CAD build for the part. Positions are in the model's coordinates, mm. Coordinates: 2 decimals unless noted, no trailing zeros. Order: outer loops, then holes, each group sorted by start corner. A loop starts at its lowest first (then second) coordinate and runs counter-clockwise, first axis right, second up. Notation, with made-up numbers: (32.5, 22.5) - (37.5, 22.5) arc R21 ccw to (37.5, 42.5) - close; hole circle Ø1 at (-25.5, 85). An arc over 180 degrees is marked (long way). Return JSON: item names as keys, results as strings.
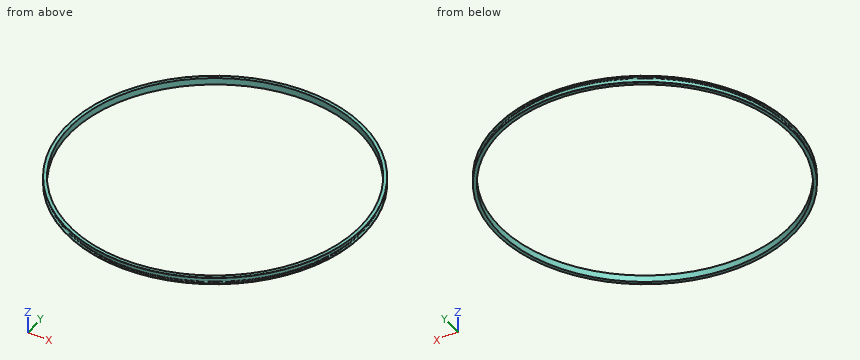
from build123d import *


with BuildPart() as part:
    # Sketch1 → Revolve1 (revolve)
    with BuildSketch(Plane(origin=(0, 0, 0), x_dir=(1, 0, 0), z_dir=(0, 1, 0))):
        with BuildLine():
            Line((850, 0), (850, 20))
            Line((850, 20), (870, 20))
            Line((870, 20), (870, 19))
            ThreePointArc((870, 19), (869.707106781, 18.292893219), (869, 18))
            Line((869, 18), (858, 18))
            ThreePointArc((858, 18), (855.171572875, 16.828427125), (854, 14))
            Line((854, 14), (854, -14))
            ThreePointArc((854, -14), (855.171572875, -16.828427125), (858, -18))
            Line((858, -18), (869, -18))
            ThreePointArc((869, -18), (869.707106781, -18.292893219), (870, -19))
            Line((870, -19), (870, -20))
            Line((870, -20), (850, -20))
            Line((850, -20), (850, 0))
        make_face()
    revolve(axis=Axis((0, 0, 0), (0, 0, -1)))


solid = part.part
Item 1: Wall check: L1, parallel to Y at x = 0, z = 10.5; L2, parallel to X at y = -485.5, z = 11. Give the ranges that are in metal, low to high. Write a range as [from, to].
Findings below:
{"L1": "y = [-854, -850], [850, 854]", "L2": "x = [-702.57, -697.7], [697.7, 702.57]"}
Item 2: Band-saw the part on A-A, the plane y = 0. List the corners of the cut face in (x, z), then the cut area to 3 significant figures.
Findings below:
{"outline": "(-870, -20) - (-850, -20) - (-850, 20) - (-870, 20) - (-870, 19) arc R1 ccw to (-869, 18) - (-858, 18) arc R4 cw to (-854, 14) - (-854, -14) arc R4 cw to (-858, -18) - (-869, -18) arc R1 ccw to (-870, -19) - close; (850, -20) - (870, -20) - (870, -19) arc R1 ccw to (869, -18) - (858, -18) arc R4 cw to (854, -14) - (854, 14) arc R4 cw to (858, 18) - (869, 18) arc R1 ccw to (870, 19) - (870, 20) - (850, 20) - close", "area": "461 mm²"}
Item 3: Band-saw the part on C-C, the plane z = -6. List the corners of the cut face in (x, y).
Findings below:
{"outline": "circle Ø1708 at (0, 0); hole circle Ø1700 at (0, 0)"}
Item 4: Drop flat-ended pins along their axis: P1, Ø1, axis at x = -378, z = 2.5, coming from the -Y side; P2, Ø5, axis at y = -380.5, z = 13.5, coming from the -X side; P3, Ø12, axis at x = -350, z = 15, coming from the -Y side. Give the stop position or say it passes through.
Findings below:
{"P1": "stops at y = -766.04", "P2": "stops at x = -765.79", "P3": "stops at y = -798.5"}
